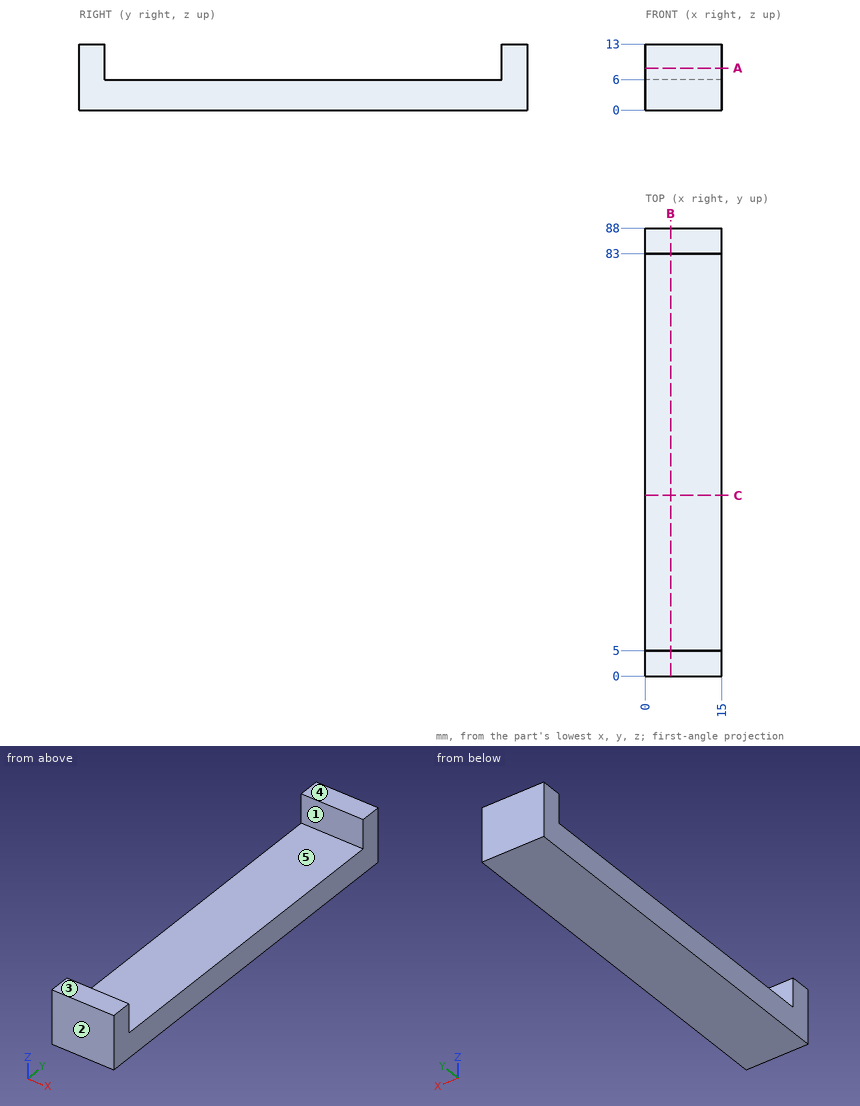
Source: three-view drawing plus pictorial views. Frame: mm from the lowest corner of the part. A direction names the side the tool comes from. Give positions to 0.01 mm unless a question says otherwise; leave off trailing zeros. Write each loop counter-clockwise with the first axis right and the second up, starting at its lowest first coordinate (ties: lowest second). Pieces come first, ordered by that corner, then holes.
(1) Mould query, pull axis Y, two halves, no side actions, for the marked faces 1, 2 and 3. Classes: released by +Y, released by -Y, zero draft, split by the parting line, or undercut.
(2) First-contact query: P1, Ø7.5, axis at x = 5.5, y = 36, coming from the +Z side. Flat tip, straight axial feed; report the tip coordinate or a pass-through.
(3) Cut plane B-B, the plane x = 5. Return loops of the section in (y, z).
(4) Access query for the marked faces 4 and 5. Directions: +Z, -Z, +X, -X, +Y, -Y. A direction counts if a zero-diameter tool reaches every point of the face in a straight line with its end or side. Return the directions, or none.
(5) Cut plane A-A, the plane z = 8.25. Return loops of the section in (x, y), then the cut area to 3 significant figures.
(6) Ray query, line 1 (Y direction, x = 6.5, z = 8.5); line 2 (Z direction, x = 12, y = 68.5). Return the intervals inside material, ascending.
(7) Cut plane C-C, the plane y = 35.5. Return loops of the section in (x, z).
Values follow:
1. face 1: undercut
1. face 2: released by -Y
1. face 3: zero draft
2. P1: stops at z = 6
3. outline: (0, 0) - (88, 0) - (88, 13) - (83, 13) - (83, 6) - (5, 6) - (5, 13) - (0, 13) - close
4. face 4: +Z, +X, -X, +Y, -Y
4. face 5: +Z, +X, -X
5. outline: (0, 0) - (15, 0) - (15, 5) - (0, 5) - close; (0, 83) - (15, 83) - (15, 88) - (0, 88) - close
5. area: 150 mm2
6. line 1: y = 0 to 5, 83 to 88
6. line 2: z = 0 to 6
7. outline: (0, 0) - (15, 0) - (15, 6) - (0, 6) - close
